Check sheet for the modelled part. Datum: model origin and axes. Units: mm. Face numbers are marked on the shaded views. A direction names the side the tool comes from. Round coordinates to 2 decimals unless told otherwise and drop trailing zeros. Loops run counter-clockwise (first coordinate to the right, second up) from the corner with the lowest first, then second, coordinate; pieces in that order, holes last. Notation, with made-up numbers: (36.5, -17) - (51.5, -17) arc R28 cw to (51.5, 21) - close; hole circle Ø6 at (28.25, 34). An arc over 180 degrees is marked (long way). Put each result on its own line as item: value.
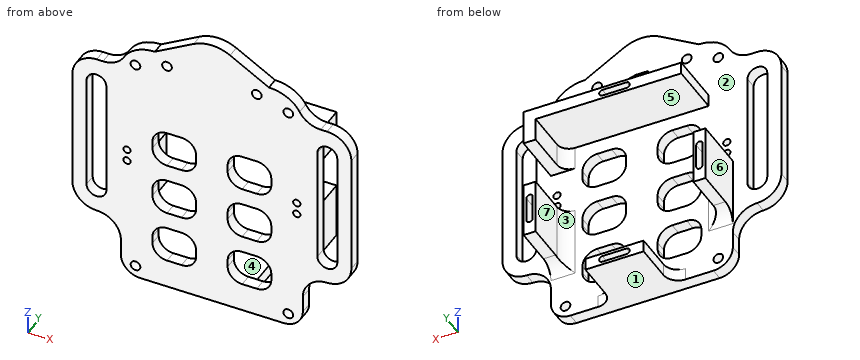
```python
from build123d import *

# Parameters (mm, degrees)
SKETCH_1_W           = 115
SKETCH_1_H           = 70
EXTRUDE_1_DEPTH      = 5
SKETCH_2_R           = 1.5
CUT_EXTRUDE_1_DEPTH  = 5
EXTRUDE_3_DEPTH      = 22
SKETCH_4_W           = 5
SKETCH_4_H           = 23
EXTRUDE_4_DEPTH      = 22
SKETCH_6_W           = 47
SKETCH_6_H           = 27
EXTRUDE_5_DEPTH      = 5
SKETCH_7_R           = 2
CUT_EXTRUDE_3_DEPTH  = 5
CHAMFER_1_SIZE       = 15
CHAMFER_1_SIZE_2     = 25.980762114
RIB_1_REACH          = 116.754
SKETCH_8_WALL_W      = 259.791929252
SKETCH_8_WALL_H      = 5
SKETCH_10_W          = 14.5
SKETCH_10_H          = 22
CUT_EXTRUDE_4_DEPTH  = 10
CUT_EXTRUDE_5_DEPTH  = 5
CUT_EXTRUDE_7_DEPTH  = 5
FILLET_1_R           = 15
EXTRUDE_7_DEPTH      = 5
SKETCH_24_W          = 75
SKETCH_24_H          = 25
EXTRUDE_10_DEPTH     = 5
SKETCH_25_R          = 2
CUT_EXTRUDE_9_DEPTH  = 5
SKETCH_26_W          = 24
SKETCH_26_H          = 5
EXTRUDE_11_DEPTH     = 22
FILLET_6_R           = 8
FILLET_START         = -1
FILLET_7_DEPTH       = 7
FILLET_7_2_DEPTH     = 5
SKETCH_28_W          = 18
SKETCH_28_H          = 15
CUT_EXTRUDE_11_DEPTH = 10
FILLET_8_R           = 6
FILLET_9_R           = 6
CUT_EXTRUDE_12_DEPTH = 10
FILLET_10_R          = 6
FILLET_11_R          = 5
CUT_EXTRUDE_13_DEPTH = 5
CUT_EXTRUDE_14_DEPTH = 5


with BuildPart() as part:
    # 草图1 → 凸台-拉伸1 (new body)
    with BuildSketch(Plane(origin=(0, 0, 0), x_dir=(1, 0, 0), z_dir=(0, 1, 0))):
        with Locations((57.5, -35)):
            Rectangle(SKETCH_1_W, SKETCH_1_H)
    extrude(amount=EXTRUDE_1_DEPTH)

    # 草图2 → 切除-拉伸1 (cut)
    with BuildSketch(Plane(origin=(0, 5, 0), x_dir=(1, 0, 0), z_dir=(0, 1, 0))):
        with Locations(Location((92.5, -27.5, 0), (0, 0, 270))):
            Circle(SKETCH_2_R)
        with Locations(Location((92.5, -32.5, 0), (0, 0, 90))):
            Circle(SKETCH_2_R)
        with Locations(Location((22.5, -32.5, 0), (0, 0, 270))):
            Circle(SKETCH_2_R)
        with Locations(Location((22.5, -27.5, 0), (0, 0, 90))):
            Circle(SKETCH_2_R)
    extrude(amount=-CUT_EXTRUDE_1_DEPTH, mode=Mode.SUBTRACT)

    # 草图3 → 凸台-拉伸3 (add)
    with BuildSketch(Plane(origin=(0, 5, 0), x_dir=(1, 0, 0), z_dir=(0, 1, 0))):
        Polygon((90, -42.5), (95, -42.5), (95, -57), (57.5, -57), (57.5, -52), (90, -52), align=None)
    extrude_3 = extrude(amount=EXTRUDE_3_DEPTH)

    # 镜向1: 凸台-拉伸3 across plane
    add(extrude_3.mirror(Plane(origin=(57.5, 27, 52), x_dir=(0, 0, 1), z_dir=(1, 0, 0))))

    # 草图4 → 凸台-拉伸4 (add)
    with BuildSketch(Plane(origin=(0, 5, 0), x_dir=(1, 0, 0), z_dir=(0, 1, 0))):
        with Locations((92.5, -11.5)):
            Rectangle(SKETCH_4_W, SKETCH_4_H)
    extrude_4 = extrude(amount=EXTRUDE_4_DEPTH)

    # 镜向2: 凸台-拉伸4 across plane
    add(extrude_4.mirror(Plane(origin=(57.5, 0, 0), x_dir=(0, 0, 1), z_dir=(1, 0, 0))))

    # 草图6 → 凸台-拉伸5 (add)
    with BuildSketch(Plane.XZ):
        with Locations((57.5, 83.5)):
            Rectangle(SKETCH_6_W, SKETCH_6_H)
    extrude(amount=-EXTRUDE_5_DEPTH)

    # 草图7 → 切除-拉伸3 (cut)
    with BuildSketch(Plane(origin=(0, 5, 0), x_dir=(1, 0, 0), z_dir=(0, 1, 0))):
        with Locations(Location((39, -77, 0), (0, 0, 270))):
            Circle(SKETCH_7_R)
        with Locations(Location((76, -77, 0), (0, 0, 90))):
            Circle(SKETCH_7_R)
    extrude(amount=-CUT_EXTRUDE_3_DEPTH, mode=Mode.SUBTRACT)

    # 倒角1
    # the kernel refuses this chamfer: 25.980762114, 15 mm, written as the material it takes off along each edge
    with BuildSketch(Plane(origin=(81, -67.214459559, 97), x_dir=(0, 0, -1), z_dir=(0, 1, 0))) as chamfer_1_piece_1:
        Polygon((CHAMFER_1_SIZE, 0), (0, CHAMFER_1_SIZE_2), (0, 0), align=None)
    extrude(amount=139.428919118, mode=Mode.SUBTRACT)
    with BuildSketch(Plane(origin=(34, -67.214459559, 97), x_dir=(1, 0, 0), z_dir=(0, 1, 0))) as chamfer_1_piece_2:
        Polygon((CHAMFER_1_SIZE_2, 0), (0, CHAMFER_1_SIZE), (0, 0), align=None)
    extrude(amount=139.428919118, mode=Mode.SUBTRACT)

    # 草图8 wall → 筋1 (add, up to next)
    with BuildSketch(Plane(origin=(57.5, 15, 67), x_dir=(0, 0.707106781187, -0.707106781187), z_dir=(0, 0.707106781187, 0.707106781187)), mode=Mode.PRIVATE) as rib_1_sk1:
        Rectangle(SKETCH_8_WALL_W, SKETCH_8_WALL_H)
    rib_1_tool1 = extrude(rib_1_sk1.sketch, amount=-RIB_1_REACH, mode=Mode.PRIVATE) - part.part
    add(rib_1_tool1.solids().sort_by_distance((57.5, 15, 67))[0])

    # 草图10 → 切除-拉伸4 (cut)
    with BuildSketch(Plane.ZY.offset(-20)):
        with Locations((49.75, 16)):
            Rectangle(SKETCH_10_W, SKETCH_10_H)
    extrude(amount=-CUT_EXTRUDE_4_DEPTH, mode=Mode.SUBTRACT)

    # 草图11 → 切除-拉伸5 (cut)
    with BuildSketch(Plane(origin=(0, 27, 0), x_dir=(1, 0, 0), z_dir=(0, 1, 0))):
        with BuildLine():
            Line((23.8, -6.5), (23.8, -16.5))
            ThreePointArc((23.8, -16.5), (22.5, -17.8), (21.2, -16.5))
            Line((21.2, -16.5), (21.2, -6.5))
            ThreePointArc((21.2, -6.5), (22.5, -5.2), (23.8, -6.5))
        make_face()
    cut_extrude_5 = extrude(amount=-CUT_EXTRUDE_5_DEPTH, mode=Mode.SUBTRACT)

    # 镜向4: 切除-拉伸5 across plane
    add(cut_extrude_5.mirror(Plane(origin=(57.5, 0, 0), x_dir=(0, 0, 1), z_dir=(1, 0, 0))), mode=Mode.SUBTRACT)

    # 草图15 → 切除-拉伸7 (cut)
    with BuildSketch(Plane.ZY.offset(-55)):
        Polygon((57, 25), (57, 10), (72, 10), align=None)
    extrude(amount=-CUT_EXTRUDE_7_DEPTH, mode=Mode.SUBTRACT)

    # 圆角1
    fillet_1_edges = [part.edges().sort_by_distance(p)[0] for p in [
        (57.5, 2.5, 95.567731326),
    ]]
    fillet(fillet_1_edges, radius=FILLET_1_R)

    # 草图18 → 凸台-拉伸7 (add)
    with BuildSketch(Plane.XZ):
        with BuildLine():
            Line((20, 70), (34, 70))
            Line((34, 70), (34, 82))
            add(Edge.make_bspline(
                [(34, 82), (20, 82), (20, 70)],
                knots=[1.570796327, 1.570796327, 1.570796327, 3.141592654, 3.141592654, 3.141592654], degree=2, weights=[1, 0.707106781, 1]))
        make_face()
    extrude_7 = extrude(amount=-EXTRUDE_7_DEPTH)

    # 镜向8: 凸台-拉伸7 across plane
    add(extrude_7.mirror(Plane(origin=(57.5, 0, 0), x_dir=(0, 0, 1), z_dir=(1, 0, 0))))

    # 草图24 → 凸台-拉伸10 (add)
    with BuildSketch(Plane.XZ):
        with Locations((57.5, -12.5)):
            Rectangle(SKETCH_24_W, SKETCH_24_H)
    extrude(amount=-EXTRUDE_10_DEPTH)

    # 草图25 → 切除-拉伸9 (cut)
    with BuildSketch(Plane(origin=(0, 5, 0), x_dir=(1, 0, 0), z_dir=(0, 1, 0))):
        with Locations(Location((89, -73, 0), (0, 0, 270))):
            Circle(SKETCH_25_R)
        with Locations(Location((89, 20, 0), (0, 0, 270))):
            Circle(SKETCH_25_R)
    cut_extrude_9 = extrude(amount=-CUT_EXTRUDE_9_DEPTH, mode=Mode.SUBTRACT)

    # 镜向11: 切除-拉伸9 across plane
    add(cut_extrude_9.mirror(Plane(origin=(57.5, 0, 0), x_dir=(0, 0, 1), z_dir=(1, 0, 0))), mode=Mode.SUBTRACT)

    # 草图26 → 凸台-拉伸11 (add)
    with BuildSketch(Plane(origin=(0, 5, 0), x_dir=(1, 0, 0), z_dir=(0, 1, 0))):
        with Locations((57.5, 22.5)):
            Rectangle(SKETCH_26_W, SKETCH_26_H)
    extrude(amount=EXTRUDE_11_DEPTH)

    # 圆角6
    fillet_6_edges = [part.edges().sort_by_distance(p)[0] for p in [
        (20, 2.5, -25),
        (95, 2.5, -25),
    ]]
    fillet(fillet_6_edges, radius=FILLET_6_R)

    # 圆角7: read off the stored shape, not the designer's step
    # 圆角7 outline → 圆角7 (cut)
    with BuildSketch(Plane(origin=(0, 0, 0), x_dir=(1, 0, 0), z_dir=(0, 1, 0)).offset(FILLET_START)):
        with BuildLine():
            ThreePointArc((105, 0), (112.071067812, -2.928932188), (115, -10))
            Line((115, -10), (115, 0))
            Line((115, 0), (105, 0))
        make_face()
        with BuildLine():
            ThreePointArc((115, -60), (112.071067812, -67.071067812), (105, -70))
            Line((105, -70), (115, -70))
            Line((115, -70), (115, -60))
        make_face()
        with BuildLine():
            Line((0, 0), (0, -10))
            ThreePointArc((0, -10), (2.928932188, -2.928932188), (10, 0))
            Line((10, 0), (0, 0))
        make_face()
        with BuildLine():
            ThreePointArc((10, -70), (2.928932188, -67.071067812), (0, -60))
            Line((0, -60), (0, -70))
            Line((0, -70), (10, -70))
        make_face()
    extrude(amount=FILLET_7_DEPTH, mode=Mode.SUBTRACT)

    # Fillet 7 2 outline → Fillet 7 2 (add)
    with BuildSketch(Plane(origin=(0, 0, 0), x_dir=(1, 0, 0), z_dir=(0, 1, 0))):
        with BuildLine():
            add(Edge.make_bspline(
                [(93.644655928, -75.150899174), (95, -72.706455982), (95, -70)],
                knots=[5.824972497, 5.824972497, 5.824972497, 6.283185307, 6.283185307, 6.283185307], degree=2, weights=[0.878968224, 0.9145609, 1]))
            ThreePointArc((93.644655928, -75.150899174), (97.315407297, -71.383416911), (102.390296052, -70))
            Line((102.390296052, -70), (95, -70))
        make_face()
        with BuildLine():
            Line((95, 0), (105, 0))
            ThreePointArc((105, 0), (97.928932188, 2.928932188), (95, 10))
            Line((95, 10), (95, 0))
        make_face()
        with BuildLine():
            Line((20, -70), (12.609703948, -70))
            ThreePointArc((12.609703948, -70), (17.684592703, -71.383416911), (21.355344072, -75.150899174))
            add(Edge.make_bspline(
                [(21.355344072, -75.150899174), (20, -72.706455982), (20, -70)],
                knots=[5.824972497, 5.824972497, 5.824972497, 6.283185307, 6.283185307, 6.283185307], degree=2, weights=[0.878968224, 0.9145609, 1]))
        make_face()
        with BuildLine():
            ThreePointArc((20, 10), (17.071067812, 2.928932188), (10, 0))
            Line((10, 0), (20, 0))
            Line((20, 0), (20, 10))
        make_face()
    extrude(amount=FILLET_7_2_DEPTH)

    # 草图28 → 切除-拉伸11 (cut)
    with BuildSketch(Plane(origin=(0, 5, 0), x_dir=(1, 0, 0), z_dir=(0, 1, 0))):
        with Locations((42, 5.5)):
            Rectangle(SKETCH_28_W, SKETCH_28_H)
        with Locations((73, 5.5)):
            Rectangle(SKETCH_28_W, SKETCH_28_H)
        with Locations((73, -16.5)):
            Rectangle(SKETCH_28_W, SKETCH_28_H)
        with Locations((73, -38.5)):
            Rectangle(SKETCH_28_W, SKETCH_28_H)
        with Locations((42, -16.5)):
            Rectangle(SKETCH_28_W, SKETCH_28_H)
        with Locations((42, -38.5)):
            Rectangle(SKETCH_28_W, SKETCH_28_H)
    extrude(amount=-CUT_EXTRUDE_11_DEPTH, mode=Mode.SUBTRACT)

    # 圆角8
    fillet_8_edges = [part.edges().sort_by_distance(p)[0] for p in [
        (82, 2.5, 46),
        (64, 2.5, 46),
        (64, 2.5, 31),
        (82, 2.5, 31),
        (82, 2.5, 24),
        (64, 2.5, 24),
        (64, 2.5, 9),
        (82, 2.5, 9),
        (82, 2.5, 2),
        (64, 2.5, 2),
        (64, 2.5, -13),
        (82, 2.5, -13),
    ]]
    fillet(fillet_8_edges, radius=FILLET_8_R)

    # 圆角9
    fillet_9_edges = [part.edges().sort_by_distance(p)[0] for p in [
        (51, 2.5, 24),
        (33, 2.5, 24),
        (33, 2.5, 9),
        (51, 2.5, 9),
        (51, 2.5, 46),
        (33, 2.5, 46),
        (33, 2.5, 31),
        (51, 2.5, 31),
        (51, 2.5, -13),
        (51, 2.5, 2),
        (33, 2.5, 2),
        (33, 2.5, -13),
    ]]
    fillet(fillet_9_edges, radius=FILLET_9_R)

    # 草图29 → 切除-拉伸12 (cut)
    with BuildSketch(Plane(origin=(0, 5, 0), x_dir=(1, 0, 0), z_dir=(0, 1, 0))):
        with BuildLine():
            Line((109.195843091, -10.700151008), (109.195843091, -58.829338195))
            ThreePointArc((109.195843091, -58.829338195), (105.102845499, -62.922335787), (101.009847907, -58.829338195))
            Line((101.009847907, -58.829338195), (101.009847907, -10.700151008))
            ThreePointArc((101.009847907, -10.700151008), (105.102845499, -6.607153417), (109.195843091, -10.700151008))
        make_face()
    cut_extrude_12 = extrude(amount=-CUT_EXTRUDE_12_DEPTH, mode=Mode.SUBTRACT)

    # 镜向16: 切除-拉伸12 across plane
    add(cut_extrude_12.mirror(Plane(origin=(57.5, 0, 0), x_dir=(0, 0, 1), z_dir=(1, 0, 0))), mode=Mode.SUBTRACT)

    # 圆角10
    fillet_10_edges = [part.edges().sort_by_distance(p)[0] for p in [
        (22.5, 5, 0),
        (92.5, 5, 0),
        (69.5, 5, -22.5),
        (45.5, 5, -22.5),
    ]]
    fillet(fillet_10_edges, radius=FILLET_10_R)

    # 圆角11
    fillet_11_edges = [part.edges().sort_by_distance(p)[0] for p in [
        (90, 5, 47.25),
        (90, 5, 8.5),
        (25, 5, 8.5),
    ]]
    fillet(fillet_11_edges, radius=FILLET_11_R)

    # 草图30 → 切除-拉伸13 (cut)
    with BuildSketch(Plane(origin=(0, 27, 0), x_dir=(1, 0, 0), z_dir=(0, 1, 0))):
        with BuildLine():
            Line((52.5, 23.8), (62.5, 23.8))
            ThreePointArc((62.5, 23.8), (63.8, 22.5), (62.5, 21.2))
            Line((62.5, 21.2), (52.5, 21.2))
            ThreePointArc((52.5, 21.2), (51.2, 22.5), (52.5, 23.8))
        make_face()
    extrude(amount=-CUT_EXTRUDE_13_DEPTH, mode=Mode.SUBTRACT)

    # 草图31 → 切除-拉伸14 (cut)
    with BuildSketch(Plane(origin=(0, 27, 0), x_dir=(1, 0, 0), z_dir=(0, 1, 0))):
        with BuildLine():
            Line((52.5, -53.2), (62.5, -53.2))
            ThreePointArc((62.5, -53.2), (63.8, -54.5), (62.5, -55.8))
            Line((62.5, -55.8), (52.5, -55.8))
            ThreePointArc((52.5, -55.8), (51.2, -54.5), (52.5, -53.2))
        make_face()
    extrude(amount=-CUT_EXTRUDE_14_DEPTH, mode=Mode.SUBTRACT)


solid = part.part
```
Item 1: Go/stop test with flat-tipped pins: pin 1 (1.5 mm diameter, centred on x = 93, y = 15, fed in from -Z); pin 2 (4 mm diameter, centred on y = 25, z = 10.5, fed in from -X); pin 3 (4 mm diameter, centred on x = 63.5, y = 23.5, fed in from +Z); pin 4 (2.5 mm diameter, centred on x = 22.5, z = 32.5, fed in from +Y). Record where each tip stops, or that it passes through.
Filled sheet:
pin 1: z = 0
pin 2: x = 20
pin 3: z = 57
pin 4: through
Item 2: Section check A-A on y = 14. Enter the section's corners in (x, z), then the cut area to 4 significant figures.
Filled sheet:
outline: (20, 0) - (25, 0) - (25, 23) - (20, 23) - close; (30, 52) - (90, 52) - (90, 42.5) - (95, 42.5) - (95, 57) - (30, 57) - close; (45.5, -25) - (69.5, -25) - (69.5, -20) - (45.5, -20) - close; (90, 0) - (95, 0) - (95, 23) - (90, 23) - close
area: 722.5 mm²
Item 3: Thickness scan on line 1 (X direction, y = 2.55, z = 27.5); line 2 (Z direction, x = 92.5, y = 23); line 3 (X direction, y = 4.75, z = -10.5). Record the ranges inside material, lowest first. Write a range as from..to.
Filled sheet:
line 1: 0..5.8, 13.99..21, 24..91, 94..101.01, 109.2..115
line 2: 0..5.2, 17.8..23, 42.5..57
line 3: 20..34.13, 49.87..65.13, 80.87..95
Item 4: Release check for a two-part mould opening along Z. For the marked faces 1, 2 and 3 record: +Z half, -Z half, draft (parallel to the pull), parting line (faces both ways), or undercut.
Filled sheet:
face 1: -Z half
face 2: undercut
face 3: draft
Item 5: Section check B-B on z = 19.5. Count the separate pieces of the cut face and the enclosed holes in it, then the cut area to 3 significant figures.
Filled sheet:
separate pieces: 5
enclosed holes: 0
area: 548 mm²
Item 6: Section check C-C on x = 106.5. Enter the section's corners in (y, z).
Filled sheet:
outline: (0, 0.11) - (5, 0.11) - (5, 6.85) - (0, 6.85) - close; (0, 62.68) - (5, 62.68) - (5, 69.89) - (0, 69.89) - close
Item 7: Tool access check on the marked faces 4, 5, 6 and 7. Record the directions out of +Z, -Z, +X, -X, +Y, -Y that give a thin tool (end or side, any length) a straight path to the whole face; none if there is none.
Filled sheet:
face 4: +X, -X, +Y
face 5: -X, +Y
face 6: +Z, -Z, -X, +Y
face 7: -Z, +Y
